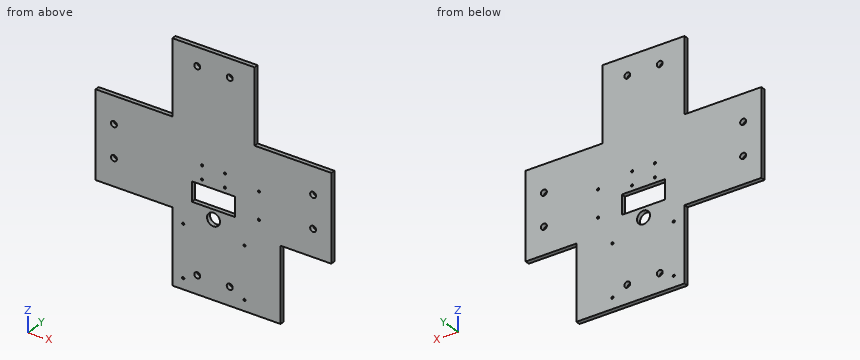
from build123d import *

# Parameters (mm, degrees)
SKETCH1_W           = 100
SKETCH1_H           = 80
BOSS_EXTRUDE1_DEPTH = 4
SKETCH2_R           = 1
CUT_EXTRUDE1_DEPTH  = 65.156059729
BOSS_EXTRUDE2_DEPTH = 4
SKETCH4_R           = 1
CUT_EXTRUDE2_DEPTH  = 4
SKETCH5_R           = 1
CUT_EXTRUDE3_DEPTH  = 4
SKETCH6_R           = 6
CUT_EXTRUDE4_DEPTH  = 95.424573073
BOSS_EXTRUDE3_DEPTH = 4
SKETCH8_R           = 2.75
CUT_EXTRUDE5_DEPTH  = 216.273272068


with BuildPart() as part:
    # Sketch1 → Boss-Extrude1 (new body)
    with BuildSketch(Plane(origin=(0, 0, 0), x_dir=(1, 0, 0), z_dir=(0, 1, 0))):
        Rectangle(SKETCH1_W, SKETCH1_H)
    extrude(amount=BOSS_EXTRUDE1_DEPTH)

    # Sketch2 → Cut-Extrude1 (cut, through all)
    with BuildSketch(Plane(origin=(0, 4, 0), x_dir=(1, 0, 0), z_dir=(0, 1, 0))):
        with Locations(Location((-40, 30, 0), (0, 0, 270))):
            Circle(SKETCH2_R)
        with Locations(Location((16.7, 30, 0), (0, 0, 270))):
            Circle(SKETCH2_R)
        with Locations(Location((16.7, -17.9, 0), (0, 0, 270))):
            Circle(SKETCH2_R)
        with Locations(Location((-40, -17.9, 0), (0, 0, 270))):
            Circle(SKETCH2_R)
    extrude(amount=-CUT_EXTRUDE1_DEPTH, mode=Mode.SUBTRACT)

    # Sketch3 → Boss-Extrude2 (add)
    with BuildSketch(Plane(origin=(0, 4, 0), x_dir=(1, 0, 0), z_dir=(0, 1, 0))):
        Polygon((7.993464363, -40), (50, -40), (50, -80), (-50, -80), (-50, -40), (-32.006535637, -40), (-32.006535637, -58), (7.993464363, -58), align=None)
    extrude(amount=-BOSS_EXTRUDE2_DEPTH)

    # Sketch4 → Cut-Extrude2 (cut)
    with BuildSketch(Plane(origin=(0, 4, 0), x_dir=(1, 0, 0), z_dir=(0, 1, 0))):
        with Locations(Location((-22.506535637, -62.75, 0), (0, 0, 270))):
            Circle(SKETCH4_R)
        with Locations(Location((-22.506535637, -75.25, 0), (0, 0, 270))):
            Circle(SKETCH4_R)
        with Locations(Location((-1.506535637, -75.25, 0), (0, 0, 270))):
            Circle(SKETCH4_R)
        with Locations(Location((-1.506535637, -62.75, 0), (0, 0, 270))):
            Circle(SKETCH4_R)
    extrude(amount=-CUT_EXTRUDE2_DEPTH, mode=Mode.SUBTRACT)

    # Sketch5 → Cut-Extrude3 (cut)
    with BuildSketch(Plane(origin=(0, 4, 0), x_dir=(1, 0, 0), z_dir=(0, 1, 0))):
        with Locations(Location((30, -45, 0), (0, 0, 270))):
            Circle(SKETCH5_R)
        with Locations(Location((30, -70, 0), (0, 0, 270))):
            Circle(SKETCH5_R)
    extrude(amount=-CUT_EXTRUDE3_DEPTH, mode=Mode.SUBTRACT)

    # Sketch6 → Cut-Extrude4 (cut, through all)
    with BuildSketch(Plane(origin=(0, 4, 0), x_dir=(1, 0, 0), z_dir=(0, 1, 0))):
        with Locations(Location((-12.006535637, -31, 0), (0, 0, 270))):
            Circle(SKETCH6_R)
    extrude(amount=-CUT_EXTRUDE4_DEPTH, mode=Mode.SUBTRACT)

    # Sketch7 → Boss-Extrude3 (add)
    with BuildSketch(Plane.XZ):
        Polygon((96.993464363, 29), (50, 29), (50, 80), (-50, 80), (-50, 29), (-121.006535637, 29), (-121.006535637, 109), (-50, 109), (-50, 178), (25.986928727, 178), (25.986928727, 109), (96.993464363, 109), align=None)
    extrude(amount=-BOSS_EXTRUDE3_DEPTH)

    # Sketch8 → Cut-Extrude5 (cut, through all)
    with BuildSketch(Plane(origin=(0, 4, 0), x_dir=(1, 0, 0), z_dir=(0, 1, 0))):
        with Locations(Location((-104.106535637, -84, 0), (0, 0, 270))):
            Circle(SKETCH8_R)
        with Locations(Location((-104.106535637, -54, 0), (0, 0, 90))):
            Circle(SKETCH8_R)
        with Locations(Location((80.093464363, -54, 0), (0, 0, 270))):
            Circle(SKETCH8_R)
        with Locations(Location((80.093464363, -84, 0), (0, 0, 90))):
            Circle(SKETCH8_R)
        with Locations(Location((-27.006535637, 23.1, 0), (0, 0, 270))):
            Circle(SKETCH8_R)
        with Locations(Location((2.993464363, 23.1, 0), (0, 0, 90))):
            Circle(SKETCH8_R)
        with Locations(Location((2.993464363, -161.1, 0), (0, 0, 270))):
            Circle(SKETCH8_R)
        with Locations(Location((-27.006535637, -161.1, 0), (0, 0, 90))):
            Circle(SKETCH8_R)
    extrude(amount=-CUT_EXTRUDE5_DEPTH, mode=Mode.SUBTRACT)


solid = part.part
Model file for the job. Use its own axes, mm. Coordinates: 2 decimals unless noted, no trailing zeros. Order: outer loops, then holes, each group sorted by start corner. A loop starts at its lowest first (then second) coordinate and runs counter-clockwise, first axis right, second up. Notation, with made-up numbers: (48.5, 4.5) -> (54.5, 4.5) arc R25 ccw to (54.5, 22.5) -> close; hole circle Ø3 at (74.5, 74). An arc over 180 degrees is marked (long way). Return JSON: item names as keys, results as strings. Group by question number.
Item 1: Wall check: line 1 along X through (y, z) = (1.9, 54); line 2 along X through (y, z) = (1.8, -23.1); line 3 along X through (y, z) = (2.5, 70). Give the ranges that are in metal, low to high. Write a range as [from, to].
Item 2: Flat gauge pin, fed straight in: P1, Ø1.2, axis at y = 2.5, z = -20, coming from the -X side. Where does the tip first touch, or does it go through?
Item 3: Saw through at D-D on y = 3.25. State how many separate pieces and enclosed holes the cut face has, then the cut area to 3 significant figures.
Item 4: Saw through at A-A on z = 84. Write the cut outline in (x, y), then the cut area to 3 significant figures.
Item 5: Saw through at B-B on x = 52.5. Write the cut outline in (y, z), then the cut area to 3 significant figures.
Item 6: Saw through at C-C on z = 161.1. Write the cut outline in (x, y).
Values found:
{
 "1": {"line 1": "x = [-121.01, -106.86], [-101.36, -32.01], [7.99, 77.34], [82.84, 96.99]", "line 2": "x = [-50, -29.76], [-24.26, 0.24], [5.74, 50]", "line 3": "x = [-121.01, 29], [31, 96.99]"},
 "2": {"P1": "stops at x = -50"},
 "3": {"separate pieces": "1", "enclosed holes": "20", "area": "28,500 mm2"},
 "4": {"outline": "(-121.01, 0) -> (-106.86, 0) -> (-106.86, 4) -> (-121.01, 4) -> close; (-101.36, 0) -> (77.34, 0) -> (77.34, 4) -> (-101.36, 4) -> close; (82.84, 0) -> (96.99, 0) -> (96.99, 4) -> (82.84, 4) -> close", "area": "828 mm2"},
 "5": {"outline": "(0, 29) -> (4, 29) -> (4, 109) -> (0, 109) -> close", "area": "320 mm2"},
 "6": {"outline": "(-50, 0) -> (-29.76, 0) -> (-29.76, 4) -> (-50, 4) -> close; (-24.26, 0) -> (0.24, 0) -> (0.24, 4) -> (-24.26, 4) -> close; (5.74, 0) -> (25.99, 0) -> (25.99, 4) -> (5.74, 4) -> close"}
}
